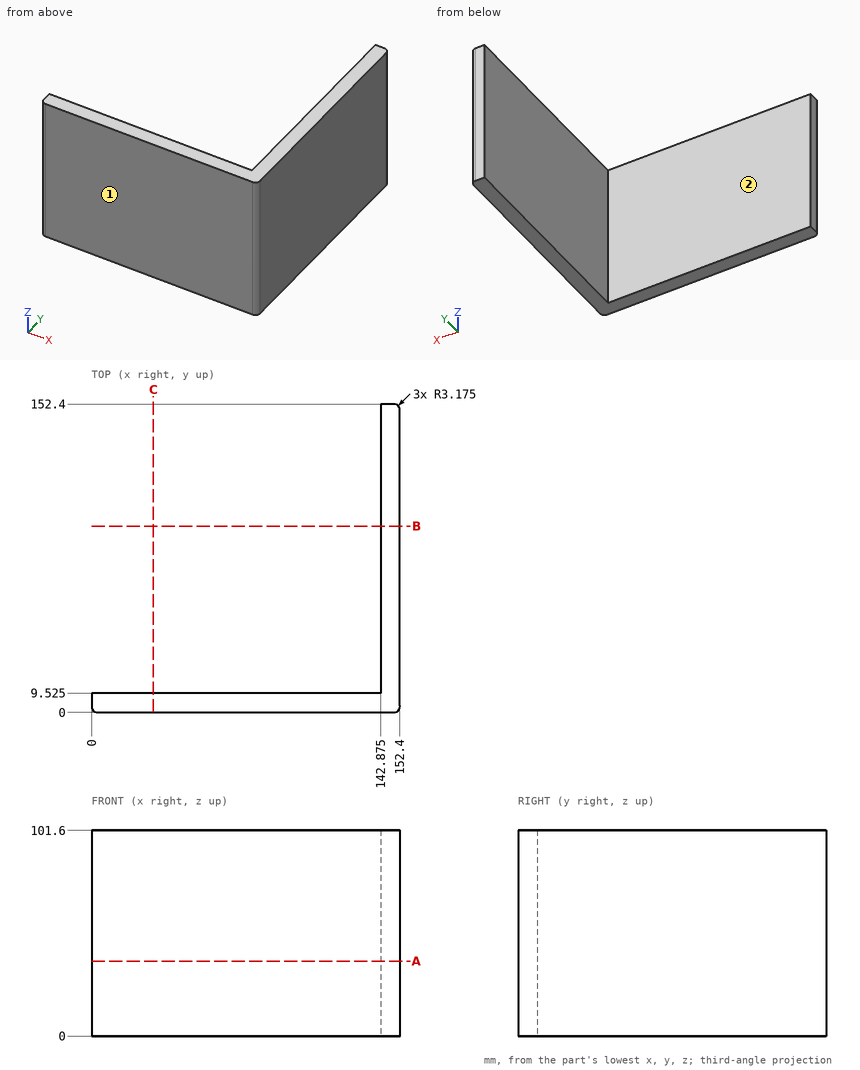
Can you work these out from the drawing? Everything is in mm from the part's minimum corner. A direction names the side the tool comes from. Round coordinates to 2 decimals unless told otherwise and drop trailing zeros. Loops run counter-clockwise (first coordinate to the right, second up) from the corner with the lowest first, then second, coordinate; pieces in that order, holes last. Notation, with made-up numbers: (85.25, 13) -> (111.25, 13) arc R8 cw to (111.25, 28) -> close; hole circle Ø6 at (71, 59.25). An arc over 180 degrees is marked (long way). Use CSV: the item, a comma, the result in double quotes.
(1) For the marked faces 1 and 2, which set-ups out of +Z, -Z, +X, -X, +Y, -Y let a thin tool reach every point of the face, with its end or its side?
Return value:
face 1,"+Z, -Z, +X, -X, -Y"
face 2,"+Z, -Z, -X, +Y"
(2) Suppose I cut it at C-C on x = 30.5. Write out the boundary of the cut face in (y, z) (3 decimals).
Return value:
outline,"(0, 0) -> (9.525, 0) -> (9.525, 101.6) -> (0, 101.6) -> close"
(3) If I drill on probe 1 along X at (y, z) = (145.5, 88) (3 decimals); probe 2 along Y at (x, z) = (142, 86.5) (3 decimals), over which ranges is the centre line in solid material (lowest first)? Write a range as [from, to].
Return value:
probe 1,"x = [142.875, 152.4]"
probe 2,"y = [0, 9.525]"
(4) Will these pins go through, and if not, where does the flat tip stop? pin 1 Ø8 at (x, z) = (118.5, 28) entering from -Y; pin 2 Ø1 at (x, z) = (137, 53.5) entering from +Y (3 decimals); pin 3 Ø4 at (y, z) = (78.5, 61) entering from -X (3 decimals).
Return value:
pin 1,"stops at y = 0"
pin 2,"stops at y = 9.525"
pin 3,"stops at x = 142.875"
(5) Suppose I cut it at A-A on z = 37. Write out the boundary of the cut face in (x, y) (3 decimals).
Return value:
outline,"(0, 3.175) arc R3.175 ccw to (3.175, 0) -> (149.225, 0) arc R3.175 ccw to (152.4, 3.175) -> (152.4, 149.225) arc R3.175 ccw to (149.225, 152.4) -> (142.875, 152.4) -> (142.875, 9.525) -> (0, 9.525) -> close"
(6) Suppose I cut it at B-B on y = 92. Write out the boundary of the cut face in (x, z) (3 decimals), plus the area to 3 significant figures.
Return value:
outline,"(142.875, 0) -> (152.4, 0) -> (152.4, 101.6) -> (142.875, 101.6) -> close"
area,"968 mm²"
